```python
from build123d import *

# Parameters (mm, degrees)
SKETCH1_W                              = 208
SKETCH1_H                              = 208
BASE_PLATE_DEPTH                       = 4
MOUNTING_HOLES_START                   = 1.5
MOUNTING_HOLES_OUTLINE_R               = 3.25
MOUNTING_HOLES_DEPTH                   = 2.5
MOUNTING_HOLES_2_OUTLINE_R             = 1.7
MOUNTING_HOLES_2_DEPTH                 = 1.5
MOUNTING_HOLES_MIRROR2_START           = 1.5
MOUNTING_HOLES_MIRROR2_COPY_1_SKETCH_R = 3.25
MOUNTING_HOLES_MIRROR2_COPY_1_DEPTH    = 2.5
MOUNTING_HOLES_MIRROR2_COPY_2_SKETCH_R = 1.7
MOUNTING_HOLES_MIRROR2_COPY_2_DEPTH    = 1.5
MOUNTING_HOLES_MIRROR2_COPY_3_SKETCH_R = 1.7
MOUNTING_HOLES_MIRROR2_COPY_3_DEPTH    = 1.5
SKETCH5_W                              = 128
SKETCH5_H                              = 4
SIDE_EXTRUSION_DEPTH                   = 14
SIDE_EXTRUSION_MIRROR2_COPY_1_SKETCH_W = 128
SIDE_EXTRUSION_MIRROR2_COPY_1_SKETCH_H = 4
SIDE_EXTRUSION_MIRROR2_COPY_1_DEPTH    = 14
EDGE_FILLETS_R                         = 3


# Read off the part's stored shape, not the designer's step: mounting_holes
with BuildPart() as part:
    # Sketch1 → base_plate (new body)
    with BuildSketch(Plane(origin=(0, 0, 0), x_dir=(1, 0, 0), z_dir=(0, 1, 0))):
        Rectangle(SKETCH1_W, SKETCH1_H)
    extrude(amount=BASE_PLATE_DEPTH)

    # mounting_holes outline → mounting_holes (cut)
    with BuildSketch(Plane(origin=(0, 0, 0), x_dir=(1, 0, 0), z_dir=(0, 1, 0)).offset(MOUNTING_HOLES_START)):
        with Locations((95, 80)):
            Circle(MOUNTING_HOLES_OUTLINE_R)
        with Locations((80, 95)):
            Circle(MOUNTING_HOLES_OUTLINE_R)
    mounting_holes = extrude(amount=MOUNTING_HOLES_DEPTH, mode=Mode.SUBTRACT)

    # mounting_holes 2 outline → mounting_holes 2 (cut)
    with BuildSketch(Plane(origin=(0, 0, 0), x_dir=(1, 0, 0), z_dir=(0, 1, 0))):
        with Locations((95, 80)):
            Circle(MOUNTING_HOLES_2_OUTLINE_R)
        with Locations((80, 95)):
            Circle(MOUNTING_HOLES_2_OUTLINE_R)
    mounting_holes_2 = extrude(amount=MOUNTING_HOLES_2_DEPTH, mode=Mode.SUBTRACT)

    # mounting_holes_mirror1: mounting_holes, mounting_holes 2 across plane
    add(mounting_holes.mirror(Plane.XY), mode=Mode.SUBTRACT)
    add(mounting_holes_2.mirror(Plane.XY), mode=Mode.SUBTRACT)

    # mounting_holes_mirror2: mounting_holes, mounting_holes 2 across plane
    add(mounting_holes.mirror(Plane(origin=(0, 0, 0), x_dir=(0, 0, 1), z_dir=(1, 0, 0))), mode=Mode.SUBTRACT)
    add(mounting_holes_2.mirror(Plane(origin=(0, 0, 0), x_dir=(0, 0, 1), z_dir=(1, 0, 0))), mode=Mode.SUBTRACT)

    # mounting_holes_mirror2 copy 1 sketch → mounting_holes_mirror2 copy 1 (cut)
    with BuildSketch(Plane(origin=(0, 0, 0), x_dir=(-1, 0, 0), z_dir=(0, 1, 0)).offset(MOUNTING_HOLES_MIRROR2_START)):
        with Locations((95, 80)):
            Circle(MOUNTING_HOLES_MIRROR2_COPY_1_SKETCH_R)
        with Locations((80, 95)):
            Circle(MOUNTING_HOLES_MIRROR2_COPY_1_SKETCH_R)
    extrude(amount=MOUNTING_HOLES_MIRROR2_COPY_1_DEPTH, mode=Mode.SUBTRACT)

    # mounting_holes_mirror2 copy 2 sketch → mounting_holes_mirror2 copy 2 (cut)
    with BuildSketch(Plane(origin=(0, 0, 0), x_dir=(-1, 0, 0), z_dir=(0, 1, 0))):
        with Locations((95, 80)):
            Circle(MOUNTING_HOLES_MIRROR2_COPY_2_SKETCH_R)
        with Locations((80, 95)):
            Circle(MOUNTING_HOLES_MIRROR2_COPY_2_SKETCH_R)
    extrude(amount=MOUNTING_HOLES_MIRROR2_COPY_2_DEPTH, mode=Mode.SUBTRACT)

    # mounting_holes_mirror2 copy 3 sketch → mounting_holes_mirror2 copy 3 (cut)
    with BuildSketch(Plane(origin=(0, 0, 0), x_dir=(-1, 0, 0), z_dir=(0, 1, 0))):
        with Locations((95, -80)):
            Circle(MOUNTING_HOLES_MIRROR2_COPY_3_SKETCH_R)
        with Locations((80, -95)):
            Circle(MOUNTING_HOLES_MIRROR2_COPY_3_SKETCH_R)
    extrude(amount=MOUNTING_HOLES_MIRROR2_COPY_3_DEPTH, mode=Mode.SUBTRACT)

    # Sketch5 → side_extrusion (add)
    with BuildSketch(Plane(origin=(0, 4, 0), x_dir=(1, 0, 0), z_dir=(0, 1, 0))):
        with Locations((0, 106)):
            Rectangle(SKETCH5_W, SKETCH5_H)
    side_extrusion = extrude(amount=-SIDE_EXTRUSION_DEPTH)

    # side_extrusion_mirror1: side_extrusion across plane
    add(side_extrusion.mirror(Plane(origin=(0, 0, 0), x_dir=(0.7071067811865476, 0, 0.7071067811865476), z_dir=(0.7071067811865477, 0, -0.7071067811865475))))

    # side_extrusion_mirror2: side_extrusion across plane
    add(side_extrusion.mirror(Plane(origin=(0, 0, 0), x_dir=(-0.7071067811865476, 0, 0.7071067811865476), z_dir=(0.7071067811865477, 0, 0.7071067811865475))))

    # side_extrusion_mirror2 copy 1 sketch → side_extrusion_mirror2 copy 1 (add)
    with BuildSketch(Plane(origin=(0, 4, 0), x_dir=(-1, 0, 0), z_dir=(0, 1, 0))):
        with Locations((0, 106)):
            Rectangle(SIDE_EXTRUSION_MIRROR2_COPY_1_SKETCH_W, SIDE_EXTRUSION_MIRROR2_COPY_1_SKETCH_H)
    extrude(amount=-SIDE_EXTRUSION_MIRROR2_COPY_1_DEPTH)

    # edge_fillets
    edge_fillets_edges = [part.edges().sort_by_distance(p)[0] for p in [
        (104, 2, 104),
        (-104, 2, 104),
        (-104, 2, -104),
        (104, 2, -104),
    ]]
    fillet(edge_fillets_edges, radius=EDGE_FILLETS_R)


solid = part.part
```
The listing builds one solid part. Answer for the finished solid, in the listing's coordinates (mm). A direction names the side the tool comes from. Round coordinates to 2 decimals unless told otherwise and drop trailing zeros. Write each loop counter-clockwise with the first axis right and the second up, starting at its lowest first coordinate (ties: lowest second). Pieces come first, ordered by that corner, then holes. Notation, with made-up numbers: (31.5, 22) -> (38.5, 22) arc R12 ccw to (38.5, 44) -> close; hole circle Ø5 at (71, 53). An arc over 180 degrees is marked (long way). Answer as a JSON object with one key per item and string values. Group by question number.
Q1. Which of the six approach directions +Z, -Z, +X, -X, +Y, -Y give full straight-line access (tool end or side, diameter ignored) to faces 4 (the face through (-1, 0, -1)), 5 (the face through (1, -5, 104)), 6 (the face through (-92.421, 2.732, -78.022)), 7 (the face through (-1, -3, -108)), 8 (the face through (104, -5, 1))?
Q2. Straight lines are drawn through the part: line 1 along Z through (x, y) = (-95, 2.1); line 2 along X through (y, z) = (1.1, 80). For each, find the intervals that lie inside material, in ascending order.
Q3. Each of these flat-tipped pins is pushed along its axis until it touches: pin 1 Ø4 at (x, z) = (85, 81) entering from -Y; pin 2 Ø4.5 at (x, y) = (91.5, 1) entering from -Z; pin 3 Ø2 at (x, z) = (-96, -81.5) entering from +Y. Where does it stop, or does it pass through?
Q4. Section A-A (y = -3.25) is taken. Write down the section's boundary in (x, z), plus the area to 3 significant figures.
Q5. Section D-D (z = -87.5) is taken. Write down the section's boundary in (x, y).
Q6. Section C-C (z = 17) is taken. Write down the section's boundary in (x, y).
Q7. Determine the mould class of faces 1 (the face through (-1, -5, -104)), 2 (the face through (-104, -5, -1)), 3 (the face through (-108, -3, -1)) for opening direction X: pulls with the +X half, pulls with the -X half, needs draft (parallel to the pull), parting line crosses it, or undercut.
Q8. Section B-B (x = 22.5) is taken. Write down the section's boundary in (y, z), plus the area to 3 significant figures.
Check values:
{
 "1": {"face 4": "-Y", "face 5": "+X, -X, -Y", "face 6": "+Y", "face 7": "-Z, +X, -X, +Y, -Y", "face 8": "+Z, -Z, -Y"},
 "2": {"line 1": "-104 to -83.25, -76.75 to 76.75, 83.25 to 104", "line 2": "-104 to -96.7, -93.3 to 93.3, 96.7 to 104"},
 "3": {"pin 1": "y = 0", "pin 2": "z = -104", "pin 3": "y = 1.5"},
 "4": {"outline": "(-108, -64) -> (-104, -64) -> (-104, 64) -> (-108, 64) -> close; (-64, -108) -> (64, -108) -> (64, -104) -> (-64, -104) -> close; (-64, 104) -> (64, 104) -> (64, 108) -> (-64, 108) -> close; (104, -64) -> (108, -64) -> (108, 64) -> (104, 64) -> close", "area": "2,050 mm^2"},
 "5": {"outline": "(-104, 0) -> (104, 0) -> (104, 4) -> (-104, 4) -> close"},
 "6": {"outline": "(-108, -10) -> (-104, -10) -> (-104, 0) -> (104, 0) -> (104, -10) -> (108, -10) -> (108, 4) -> (-108, 4) -> close"},
 "7": {"face 1": "needs draft", "face 2": "undercut", "face 3": "pulls with the -X half"},
 "8": {"outline": "(-10, -108) -> (4, -108) -> (4, 108) -> (-10, 108) -> (-10, 104) -> (0, 104) -> (0, -104) -> (-10, -104) -> close", "area": "944 mm^2"}
}
